For this review, take the finished solid that the model builds, in its own axes (mm). A direction names the side the tool comes from. Round coordinates to 2 decimals unless told otherwise and drop trailing zeros. Write each loop counter-clockwise with the first axis right and the second up, starting at its lowest first coordinate (ties: lowest second). Pieces come first, ordered by that corner, then holes. Notation, with made-up numbers: (52, 34.5) - (100, 34.5) arc R19 ccw to (100, 64.5) - close; hole circle Ø7 at (-1, 80). An arc over 180 degrees is marked (long way). One line per item, written item: value. Start each with the question number.
Q1. Mouldability with a two-part tool opening along Y and no side actions: class faces 4 (the face through (19.63, 19.7, -29.16)), 5 (the face through (-28.2, 0, -27)), 6 (the face through (-23.9, 26.05, -2.46)), 7 (the face through (-27.63, -17.6, -29.84)) as +Y half, -Y half, draft (parallel to the pull), parting line (faces both ways), or undercut.
Q2. For probe 1 along Y at (x, z) = (-23.57, -3.95); probe 2 along X at (y, z) = (23, -1), list the stretches that pass through material, from the lowest coordinate up.
Q3. Clearance check with flat-ended pins moving along their axes: pin 1 Ø3.5 at (y, z) = (-25, -22) entering from -X; pin 2 Ø3.5 at (x, z) = (-25, -18) entering from +Y; pin 3 Ø1.5 at (x, z) = (-24, -32.5) entering from -Y; pin 4 Ø19 at (x, y) = (2.5, -8.5) entering from +Z. State where each tip first meets the part, or that it passes through.
Q4. Add section A-A on x = 0. Write out the cut boundary in (y, z) (3 decimals).
Q5. Tool access review of faces 1 (the face through (-25, 18.2, -29)), 2 (the face through (27.63, -17.6, -29.84)), 3 (the face through (-24.68, -17.6, -55.43)): name each direction out of +Z, -Z, +X, -X, +Y, -Y from which nothing blocks a thin tool from reaching the whole face with its end or side.
Q6. Add section B-B on z = -15. Write out the cut boundary in (x, y), and give its area (3 significant figures).
Q7. Add section D-D on x = -7.5. Write out the cut boundary in (y, z), and give its area (3 significant figures).
```python
from build123d import *

# Parameters (mm, degrees)
SKETCH1_R           = 2.5
BOSS_EXTRUDE2_DEPTH = 56
CUT_EXTRUDE1_DEPTH  = 65.741640387
SKETCH3_R           = 19.05
BOSS_EXTRUDE3_DEPTH = 1.6
SKETCH4_R           = 3.175
BOSS_EXTRUDE4_DEPTH = 21
FILLET1_R           = 2


with BuildPart() as part:
    # Sketch1 → Boss-Extrude2 (new body)
    with BuildSketch(Plane.XY):
        with BuildLine():
            Line((-25.2, 28.2), (25.2, 28.2))
            ThreePointArc((25.2, 28.2), (27.321320344, 27.321320344), (28.2, 25.2))
            Line((28.2, 25.2), (28.2, -25.2))
            ThreePointArc((28.2, -25.2), (27.321320344, -27.321320344), (25.2, -28.2))
            Line((25.2, -28.2), (-25.2, -28.2))
            ThreePointArc((-25.2, -28.2), (-27.321320344, -27.321320344), (-28.2, -25.2))
            Line((-28.2, -25.2), (-28.2, 25.2))
            ThreePointArc((-28.2, 25.2), (-27.321320344, 27.321320344), (-25.2, 28.2))
        make_face()
        with Locations((23.57, 23.57)):
            Circle(SKETCH1_R, mode=Mode.SUBTRACT)
        with Locations((-23.57, 23.57)):
            Circle(SKETCH1_R, mode=Mode.SUBTRACT)
        with Locations((-23.57, -23.57)):
            Circle(SKETCH1_R, mode=Mode.SUBTRACT)
        with Locations((23.57, -23.57)):
            Circle(SKETCH1_R, mode=Mode.SUBTRACT)
    extrude(amount=-BOSS_EXTRUDE2_DEPTH)

    # Sketch2 → Cut-Extrude1 (cut, through all)
    with BuildSketch(Plane.XY.offset(-5)):
        with BuildLine():
            Line((18.2, 28.2), (18.2, 23.2))
            ThreePointArc((18.2, 23.2), (19.664466094, 19.664466094), (23.2, 18.2))
            Line((23.2, 18.2), (28.2, 18.2))
            Line((28.2, 18.2), (28.2, 25.2))
            ThreePointArc((28.2, 25.2), (27.321320344, 27.321320344), (25.2, 28.2))
            Line((25.2, 28.2), (18.2, 28.2))
        make_face()
        with BuildLine():
            Line((-28.2, 18.2), (-28.2, 25.2))
            ThreePointArc((-28.2, 25.2), (-27.321320344, 27.321320344), (-25.2, 28.2))
            Line((-25.2, 28.2), (-18.2, 28.2))
            Line((-18.2, 28.2), (-18.2, 23.2))
            ThreePointArc((-18.2, 23.2), (-19.664466094, 19.664466094), (-23.2, 18.2))
            Line((-23.2, 18.2), (-28.2, 18.2))
        make_face()
        with BuildLine():
            Line((-18.2, -28.2), (-18.2, -23.2))
            ThreePointArc((-18.2, -23.2), (-19.664466094, -19.664466094), (-23.2, -18.2))
            Line((-23.2, -18.2), (-28.2, -18.2))
            Line((-28.2, -18.2), (-28.2, -25.2))
            ThreePointArc((-28.2, -25.2), (-27.321320344, -27.321320344), (-25.2, -28.2))
            Line((-25.2, -28.2), (-18.2, -28.2))
        make_face()
        with BuildLine():
            Line((28.2, -18.2), (28.2, -25.2))
            ThreePointArc((28.2, -25.2), (27.321320344, -27.321320344), (25.2, -28.2))
            Line((25.2, -28.2), (18.2, -28.2))
            Line((18.2, -28.2), (18.2, -23.2))
            ThreePointArc((18.2, -23.2), (19.664466094, -19.664466094), (23.2, -18.2))
            Line((23.2, -18.2), (28.2, -18.2))
        make_face()
    extrude(amount=-CUT_EXTRUDE1_DEPTH, mode=Mode.SUBTRACT)

    # Sketch3 → Boss-Extrude3 (add)
    with BuildSketch(Plane.XY):
        Circle(SKETCH3_R)
    extrude(amount=BOSS_EXTRUDE3_DEPTH)

    # Sketch4 → Boss-Extrude4 (add)
    with BuildSketch(Plane.XY):
        with Locations(Location((0, 0, 0), (0, 0, 180))):
            Circle(SKETCH4_R)
    extrude(amount=BOSS_EXTRUDE4_DEPTH)

    # Fillet1
    fillet1_edges = [part.edges().sort_by_distance(p)[0] for p in [
        (-25.7, -18.2, -56),
        (-28.2, -18.2, -30.5),
        (-19.664466094, -19.664466094, -56),
        (-18.2, -25.7, -56),
        (-18.2, -28.2, -30.5),
        (0, 28.2, -56),
        (18.2, 28.2, -30.5),
        (25.7, 18.2, -56),
        (28.2, 18.2, -30.5),
        (19.664466094, 19.664466094, -56),
        (18.2, 25.7, -56),
        (-28.2, 0, -56),
        (-18.2, 25.7, -56),
        (-18.2, 28.2, -30.5),
        (-19.664466094, 19.664466094, -56),
        (-25.7, 18.2, -56),
        (-28.2, 18.2, -30.5),
        (28.2, 0, -56),
        (18.2, -25.7, -56),
        (18.2, -28.2, -30.5),
        (19.664466094, -19.664466094, -56),
        (25.7, -18.2, -56),
        (28.2, -18.2, -30.5),
        (0, -28.2, -56),
    ]]
    fillet(fillet1_edges, radius=FILLET1_R)


solid = part.part
```
Result set:
1. face 4: +Y half
1. face 5: draft
1. face 6: undercut
1. face 7: -Y half
2. probe 1: y = -28.2 to -26.07, -21.07 to 21.07, 26.07 to 28.2
2. probe 2: x = -28.2 to -26, -21.14 to 21.14, 26 to 28.2
3. pin 1: stops at x = -18.2
3. pin 2: stops at y = 18.2
3. pin 3: stops at y = -18.2
3. pin 4: stops at z = 21
4. outline: (-28.2, -54) arc R2 ccw to (-26.2, -56) - (26.2, -56) arc R2 ccw to (28.2, -54) - (28.2, 0) - (19.05, 0) - (19.05, 1.6) - (3.175, 1.6) - (3.175, 21) - (-3.175, 21) - (-3.175, 1.6) - (-19.05, 1.6) - (-19.05, 0) - (-28.2, 0) - close
5. face 1: -Z, -X, +Y
5. face 2: -Z, +X, -Y
5. face 3: -Z, -X, -Y
6. outline: (-28.2, -16.2) arc R2 ccw to (-26.2, -18.2) - (-23.2, -18.2) arc R5 cw to (-18.2, -23.2) - (-18.2, -26.2) arc R2 ccw to (-16.2, -28.2) - (16.2, -28.2) arc R2 ccw to (18.2, -26.2) - (18.2, -23.2) arc R5 cw to (23.2, -18.2) - (26.2, -18.2) arc R2 ccw to (28.2, -16.2) - (28.2, 16.2) arc R2 ccw to (26.2, 18.2) - (23.2, 18.2) arc R5 cw to (18.2, 23.2) - (18.2, 26.2) arc R2 ccw to (16.2, 28.2) - (-16.2, 28.2) arc R2 ccw to (-18.2, 26.2) - (-18.2, 23.2) arc R5 cw to (-23.2, 18.2) - (-26.2, 18.2) arc R2 ccw to (-28.2, 16.2) - close
6. area: 2,800 mm^2
7. outline: (-28.2, -54) arc R2 ccw to (-26.2, -56) - (26.2, -56) arc R2 ccw to (28.2, -54) - (28.2, 0) - (17.51, 0) - (17.51, 1.6) - (-17.51, 1.6) - (-17.51, 0) - (-28.2, 0) - close
7. area: 3,210 mm^2
